Part model, mm, in its own coordinate system. A direction names the side the tool comes from. Round coordinates to 2 decimals unless told otherwise and drop trailing zeros. Write each loop counter-clockwise with the first axis right and the second up, starting at its lowest first coordinate (ties: lowest second). Pieces come first, ordered by that corner, then holes.
1) Drill centre lines: L1, parallel to Y at x = -11, z = 27; L2, parallel to X at y = 4.5, z = -21; L3, parallel to Y at x = -10.5, z = -21. Where is each one in solid material? Low to high.
2) Pull direction Z, two halves, no side cores. Call faces 1 (the flat face through (-9.59, 0, 24)), 2 (the flat face through (-7.05, 0, 27)), 3 (the flat face through (-11, 0, 30.797)), 4 (the flat face through (-12.13, 0, 24)): +Z half, -Z half, draft (parallel to the pull), parting line (faces both ways), or undercut.
3) Flat gauge pins, fed straight in: pin 1 (3 mm diameter, centred on x = -8.5, y = -0.5, fed in from +Z); pin 2 (4 mm diameter, centred on x = -11, z = 27.5, fed in from -Y); pin 3 (2 mm diameter, centred on y = 0.5, z = 29, fed in from -X); pin 4 (12 mm diameter, centred on x = 1.5, y = -13, fed in from +Z). Where does each tip first touch, or does it go through?
4) Which spindle directions (+Z, -Z, +X, -X, +Y, -Y) get a long thin tool onto all of the face, cutting with end or side? Do faces 5 (the flat face through (-11, 1.27, 27)), 6 (the conical face through (-0.518, -4.288, 17.153)), 7 (the flat face through (-8, 0, 25.717)), 8 (the flat face through (-9.59, 0, 30)). Say none if no direction does.
5) Saw through at C-C on z = 9. Write the cut outline in (x, y).
6) Saw through at B-B on z = -12. Write the cut outline in (x, y), and give its area (3 significant figures).
```python
from build123d import *

# Parameters (mm, degrees)
F2_DEPTH = 1.27


with BuildPart() as f1:
    # F0 (on Front) → F1 (revolve)
    with BuildSketch(Plane.XZ):
        with BuildLine():
            Line((-10.8595, 23.176616), (-10.8595, -28.108846))
            Line((-10.8595, -28.108846), (5.828938, -28.108846))
            Line((5.828938, -28.108846), (6.631959, -22.209617))
            ThreePointArc((6.631959, -22.209617), (7.2054, -20.8997), (6.279642, -19.809889))
            ThreePointArc((6.279642, -19.809889), (4.337177, -18.849044), (2.768878, -17.35344))
            ThreePointArc((2.768878, -17.35344), (-2.043012, -7.543205), (-2.61231, 3.368755))
            ThreePointArc((-2.61231, 3.368755), (-1.297535, 6.30196), (1.343976, 8.133555))
            Line((1.343976, 8.133555), (3.905977, 15.989157))
            Line((3.905977, 15.989157), (0.153749, 17.212897))
            Line((0.153749, 17.212897), (1.144844, 20.251788))
            Line((1.144844, 20.251788), (-7.823259, 23.176616))
            Line((-7.823259, 23.176616), (-9.5895, 23.176616))
            Line((-9.5895, 23.176616), (-10.8595, 23.176616))
        make_face()
    revolve(axis=Axis((-10.8595, 0, -2.466115), (0, 0, 1)))

    # F0 (on Front) → F2 (join, symmetric)
    with BuildSketch(Plane.XZ):
        Polygon((-12.1295, 23.176616), (-10.8595, 23.176616), (-9.5895, 23.176616), (-9.5895, 25.716616), (-7.0495, 25.716616), (-7.0495, 28.256616), (-9.5895, 28.256616), (-9.5895, 30.796616), (-10.8595, 30.796616), (-12.1295, 30.796616), (-12.1295, 28.256616), (-14.6695, 28.256616), (-14.6695, 25.716616), (-12.1295, 25.716616), align=None)
    extrude(amount=F2_DEPTH, both=True)


solid = f1.part
```
Completed:
1. L1: y = -1.27 to 1.27
1. L2: x = -28.37 to 6.65
1. L3: y = -18.07 to 18.07
2. face 1: undercut
2. face 2: draft
2. face 3: +Z half
2. face 4: undercut
3. pin 1: stops at z = 30.8
3. pin 2: stops at y = -1.27
3. pin 3: stops at x = -14.67
3. pin 4: stops at z = 20.27
4. face 5: +Z, +X, -X, +Y
4. face 6: none
4. face 7: +X, +Y, -Y
4. face 8: +Z, +X, +Y, -Y
5. outline: circle Ø24.97 at (-10.86, 0)
6. outline: circle Ø20.8 at (-10.86, 0)
6. area: 340 mm2
